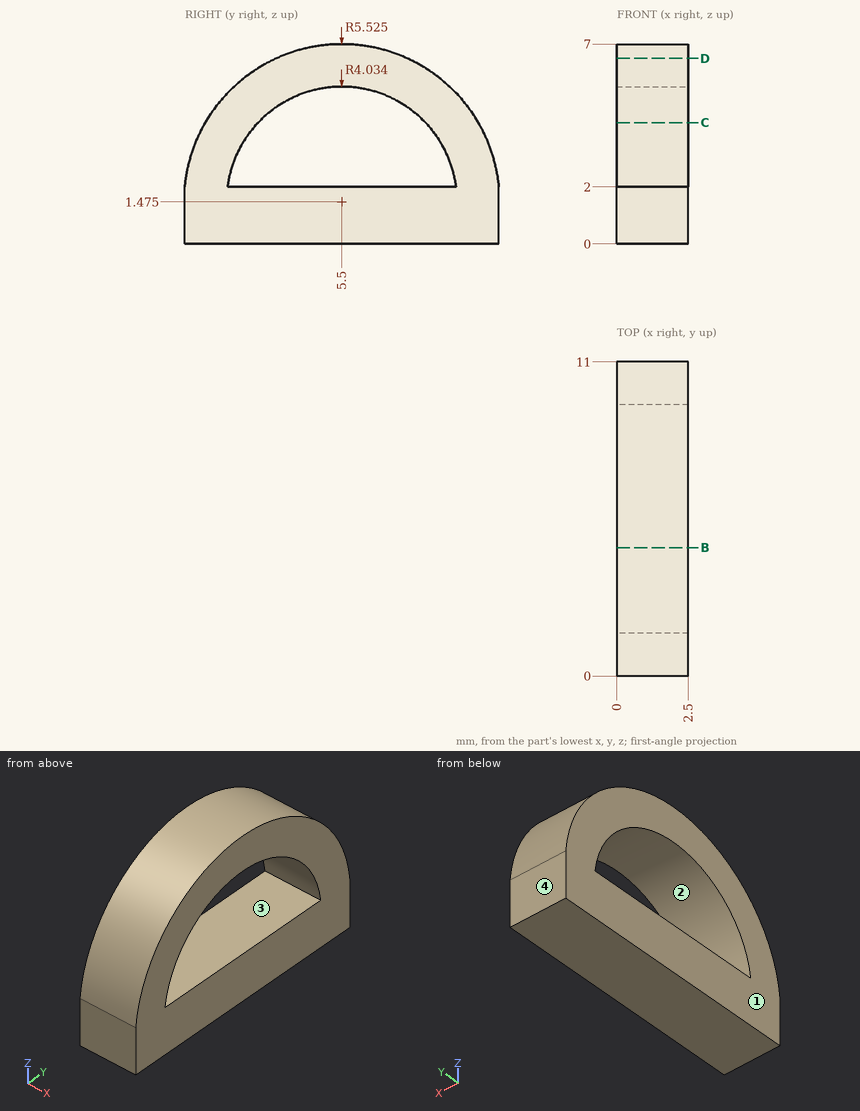
Design review of the part shown in the three views and the two pictorial views. Dimensions are in mm from the part's minimum x, y and z. Round coordinates to 2 decimals unless told otherwise and drop trailing zeros. Order: outer loops, then holes, each group sorted by start corner. A loop starts at its lowest first (then second) coordinate and runs counter-clockwise, first axis right, second up. Notation, with made-up numbers: (52, 72) - (91, 72) arc R11 ccw to (91, 81) - close; hole circle Ø7 at (50, -1). An arc over 180 degrees is marked (long way). One line per question, with ' | ' between items.
Item 1: Take a section at C-C, the plane z = 4.25. Write out the cut boundary in (x, y).
Checks:
outline: (0, 0.72) - (2.5, 0.72) - (2.5, 2.57) - (0, 2.57) - close; (0, 8.43) - (2.5, 8.43) - (2.5, 10.28) - (0, 10.28) - close
Item 2: Take a section at D-D, the plane z = 6.5. Write out the cut boundary in (x, y).
Checks:
outline: (0, 3.2) - (2.5, 3.2) - (2.5, 7.8) - (0, 7.8) - close
Item 3: For P1, Ø1.5, axis at x = 1.5, z = 4.5, coming from the +Y side (1 decimal), flat-tipped, find the tip position at first contact; note if it passes through.
Checks:
P1: y = 10.5
Item 4: Wall thickness on line 1 (Y direction, x = 0.7, z = 3.25); line 2 (Y direction, x = 1.8, z = 5) (1 decimal); line 3 (Z direction, x = 0.35, y = 8.5) (1 decimal): over which ranges is each line inside the solid? List them lowest first. Write a range as [from, to].
Checks:
line 1: [0.27, 1.88], [9.12, 10.73] | line 2: [1.2, 3.5], [7.5, 9.8] | line 3: [0, 2], [4.2, 6.1]
Item 5: Draft analysis for pull direction Y (two halves, no side actions). For the marked faces 1, 2, 3 and 4, state which applies: +Y half, -Y half, draft (parallel to the pull), parting line (faces both ways), or undercut.
Checks:
face 1: draft | face 2: undercut | face 3: undercut | face 4: +Y half
Item 6: Take a section at B-B, the plane y = 4.5. Write out the cut boundary in (x, z).
Checks:
outline: (0, 0) - (2.5, 0) - (2.5, 2) - (0, 2) - close; (0, 5.38) - (2.5, 5.38) - (2.5, 6.91) - (0, 6.91) - close
